For this review, take the finished solid that the model builds, in its own axes (mm). A direction names the side the tool comes from. Coordinates: 2 decimals unless noted, no trailing zeros. Write each loop counter-clockwise with the first axis right and the second up, starting at its lowest first coordinate (ties: lowest second). Pieces come first, ordered by that corner, then holes. Notation, with made-up numbers: (73, 59) - (90, 59) arc R16 ccw to (90, 64) - close; hole circle Ø4 at (35, 37). An arc over 180 degrees is marked (long way). Write each question's results on one line, items separated by ' | '.
from build123d import *

# Parameters (mm, degrees)
SKETCH1_W           = 25.4
SKETCH1_H           = 25.4
SKETCH1_W_2         = 22.225
SKETCH1_H_2         = 22.225
BOSS_EXTRUDE1_DEPTH = 533.4
SKETCH2_W           = 6.35
SKETCH2_H           = 12.7
CUT_EXTRUDE1_DEPTH  = 25.4
SKETCH3_R           = 3.175
CUT_EXTRUDE2_DEPTH  = 25.4
SKETCH4_R           = 3.175
CUT_EXTRUDE3_DEPTH  = 25.4


with BuildPart() as part:
    # Sketch1 → Boss-Extrude1 (new body)
    with BuildSketch(Plane(origin=(0, 0, 0), x_dir=(1, 0, 0), z_dir=(0, 1, 0))):
        Rectangle(SKETCH1_W, SKETCH1_H)
        Rectangle(SKETCH1_W_2, SKETCH1_H_2, mode=Mode.SUBTRACT)
    extrude(amount=BOSS_EXTRUDE1_DEPTH)

    # Sketch2 → Cut-Extrude1 (cut)
    with BuildSketch(Plane.XY.offset(12.7)):
        with Locations((-9.525, 6.35)):
            Rectangle(SKETCH2_W, SKETCH2_H)
    extrude(amount=-CUT_EXTRUDE1_DEPTH, mode=Mode.SUBTRACT)

    # Sketch3 → Cut-Extrude2 (cut)
    with BuildSketch(Plane.XY.offset(12.7)):
        with Locations((0, 6.35)):
            Circle(SKETCH3_R)
    extrude(amount=-CUT_EXTRUDE2_DEPTH, mode=Mode.SUBTRACT)

    # Sketch4 → Cut-Extrude3 (cut)
    with BuildSketch(Plane(origin=(12.7, 0, 0), x_dir=(0, 0, -1), z_dir=(1, 0, 0))):
        with Locations((0, 444.5)):
            Circle(SKETCH4_R)
    extrude(amount=-CUT_EXTRUDE3_DEPTH, mode=Mode.SUBTRACT)


solid = part.part
Q1. Take a section at A-A on y = 149.5. State the section outline as (x, z) points, plus the area to 3 significant figures.
Results found:
outline: (-12.7, -12.7) - (12.7, -12.7) - (12.7, 12.7) - (-12.7, 12.7) - close; hole (-11.11, -11.11) - (11.11, -11.11) - (11.11, 11.11) - (-11.11, 11.11) - close | area: 151 mm2
Q2. Mouldability with a two-part tool opening along X and no side actions: class faces 3 (the face through (-11.3, 533.4, -0.1)), 4 (the face through (11.112, 263, 0)), 5 (the face through (12.7, 263, 0)) as pulls with the +X half, pulls with the -X half, needs draft (parallel to the pull), parting line crosses it, or undercut.
Results found:
face 3: needs draft | face 4: undercut | face 5: pulls with the +X half
Q3. For pin 1 (7.5 mm diameter, centred on x = 0, y = 6.35, fed in from -Z); pin 2 (1.3 mm diameter, centred on y = 4.5, z = -12, fed in from -X); pin 3 (1.9 mm diameter, centred on x = -10.5, z = 2, fed in from -Y), all flat-tipped, find the tip position at first contact; note any pin that passes through.
Results found:
pin 1: z = -12.7 | pin 2: x = -6.35 | pin 3: y = 12.7
Q4. Wall thickness on line 1 along Y through (x, z) = (0, 11.75) (3 decimals); line 2 along Y through (x, z) = (-12, 0) (3 decimals); line 3 along Z through (x, y) = (11.7, 444.5) (3 decimals): over which ranges is each line inside the solid? List them lowest first. Write a range as from..to.
Results found:
line 1: 0..3.175, 9.525..533.4 | line 2: 12.7..441.325, 447.675..533.4 | line 3: -12.7..-3.175, 3.175..12.7
Q5. For faces 1 (the face through (-11.112, 269, 0)), 2 (the face through (-12.7, 269, 0)), list the 3-axis set-ups (+Z, -Z, +X, -X, +Y, -Y) from which the entire face can be reached by the end or side of a thin tool; tool diameter is ignored.
Results found:
face 1: +Y, -Y | face 2: +Z, -Z, -X, +Y, -Y
